Autodesk Inventor part; units mm, degrees
ref_plane "YZ Plane" through (0, 0, 0) normal (1, 0, 0) x (0, 1, 0)
ref_plane "XZ Plane" through (0, 0, 0) normal (0, 1, 0) x (-1, 0, 0)
ref_plane "XY Plane" through (0, 0, 0) normal (0, 0, 1) x (1, 0, 0)
sketch "Sketch1" plane through (0, 0, 0) normal (0, 0, 1) x (1, 0, 0)
  line L0 (6.4, 0) -> (7.6, 0)
  line L1 (12, -2.5403) -> (12, -5.8)
  line L2 (7.25, -6.4) -> (5, -6.4)
  line L3 (5, -6.4) -> (5, -16.4)
  line L4 (5, -16.4) -> (0, -16.4)
  line L5 (0, -16.4) -> (0, 0)
  line L6 (7.25, -6.4) -> (7.25, -5.8)
  line L7 (7.25, -5.8) -> (12, -5.8)
  line L8 (0, -1.28) -> (6.1, -1.28)
  line L9 (6.4, -0.98) -> (6.4, 0)
  line L10 (7.6, 0) -> (12, -2.5403)
  arc A0 (6.1, -1.28) -> (6.4, -0.98) centre (6.1, -0.98) ccw
  dimension "d0" = 24
  dimension "d1" = 10
  dimension "d3" = 10
  dimension "d4" = 14.5
  dimension "d5" = 0.6
  dimension "d26" = 15.2
  dimension "d27" = 30
  dimension "d28" = 12.8
  dimension "d29" = 1.28
  dimension "d30" = 0.3
  dimension "d31" = 6.4
revolve "Revolution1" add sketch "Sketch1" angle 360 about axis through (0, -16.4, 0) along (0, 1, 0)
sketch "Sketch2" plane through (0, 0, 0) normal (0, 1, 0) x (1, 0, 0)
  line L0 (0, -9.2376) -> (-8, -4.6188)
  line L1 (-8, -4.6188) -> (-8, 4.6188)
  line L2 (-8, 4.6188) -> (0, 9.2376)
  line L3 (0, 9.2376) -> (8, 4.6188)
  line L4 (8, 4.6188) -> (8, -4.6188)
  line L5 (8, -4.6188) -> (0, -9.2376)
  circle A0 centre (0, 0) radius 12
  point P0 (0, 0)
  point P1 (0, 0)
  dimension "d32" = 16
extrude "Extrusion1" cut sketch "Sketch2" against normal blind 5.8
thread "Thread1"
chamfer "Chamfer1" distance 0.8333 angle 45 1 edges at (-5, -16.4, 0)
equation "\"d0\" = 1.5 * S_"
equation "\"d1\" = d1_"
equation "\"d3\" = L"
equation "\"d4\" = dw"
equation "\"d5\" = hw"
equation "\"d26\" = 0.95 * S_"
equation "\"d28\" = 0.8 * S_"
equation "\"d29\" = 0.2 * k"
equation "\"d31\" = k"
equation "\"d14\" = b"
equation "\"d16\" = 0.0833333 * d"
equation "\"d32\" = S_"
equation "\"d33\" = k - hw"
equation "\"d1_\" = 10"
equation "\"S_\" = 16"
equation "\"k\" = 6.4"
equation "\"e\" = 17.6"
equation "\"L\" = 10"
equation "\"b\" = 8"
equation "\"Grip_Length\" = 2"
equation "\"dw\" = 14.5"
equation "\"hw\" = 0.6"
properties part number "Bolt 4A M10-6g×10(S16) GOST 7798-70" material "Steel, Mild"
Read the model definition and answer for the solid it produces. Units are mm, in the model's axes. A direction names the side the tool comes from. Coordinates: 2 decimals unless noted, no trailing zeros. Loops run counter-clockwise (first coordinate to the right, second up) from the corner with the lowest first, then second, coordinate; pieces in that order, holes last. Notation, with made-up numbers: (65.25, -23) -> (80.25, -23) arc R12 ccw to (80.25, -14) -> close; hole circle Ø5 at (33, -1.75). An arc over 180 degrees is marked (long way). Write item = value, one per line. Start each with the question number.
1) Given P1, Ø3.5, axis at x = 0, z = 2, coming from the +Y side; P2, Ø3, axis at y = -11, z = 2.5, coming from the -X side; P3, Ø1, axis at x = 4, y = -13, coming from the -Z side, each flat-ended and moving along its own axis, determine where each tip first touches the part or whether it passes through.
2) The part is cut by section B-B, the plane y = -5.5. Determine the outline of the cut face in (x, z), plus the area to 3 significant figures.
3) Find the intervals of material crossed by L1, parallel to X at y = -0.3, z = 0; L2, parallel to Y at x = 2.25, z = -2.25; L3, parallel to X at y = -6, z = 0.25, in increasing order. Write a range as from..to.
4) The part is cut by section A-A, the plane z = 0. Determine the outline of the cut face in (x, y), plus the area to 3 significant figures.
5) The part is cut by section C-C, the plane y = -14. Determine the outline of the cut face in (x, z).
6) The mould has two halves that part along X. Classify faces 1 (the face through (3.35, -6.1, 6.43)), 2 (the face through (-8, -3, 0)), 3 (the face through (-5.08, -0.48, 3.89)): pulls with the +X half, pulls with the -X half, needs draft (parallel to the pull), parting line crosses it, or undercut.
7) For faces 4 (the face through (-5, -5.8, -6)), 5 (the face through (3.944, -2.976, -6.961)), 6 (the face through (0, -1.28, 0)), determine the directions among +Z, -Z, +X, -X, +Y, -Y from which every point of the face is accessible in a straight line to the end or side of a thin tool.
Result:
q1.P1 = -1.28
q1.P2 = -4.9
q1.P3 = -3.57
q2.outline = (-8, -4.62) -> (0, -9.24) -> (8, -4.62) -> (8, 4.62) -> (0, 9.24) -> (-8, 4.62) -> close
q2.area = 222 mm²
q3.L1 = -8..-6.4, 6.4..8
q3.L2 = -16.4..-1.28
q3.L3 = -7.25..7.25
q4.outline = (-8, -5.8) -> (-7.25, -5.8) -> (-7.25, -6.4) -> (-5, -6.4) -> (-5, -15.57) -> (-4.17, -16.4) -> (4.17, -16.4) -> (5, -15.57) -> (5, -6.4) -> (7.25, -6.4) -> (7.25, -5.8) -> (8, -5.8) -> (8, -0.23) -> (7.6, 0) -> (6.4, 0) -> (6.4, -0.98) arc R0.3 cw to (6.1, -1.28) -> (-6.1, -1.28) arc R0.3 cw to (-6.4, -0.98) -> (-6.4, 0) -> (-7.6, 0) -> (-8, -0.23) -> close
q4.area = 184 mm²
q5.outline = circle Ø10 at (0, 0)
q6.face_1 = parting line crosses it
q6.face_2 = pulls with the -X half
q6.face_3 = undercut
q7.face_4 = -Y
q7.face_5 = -Z, +X, +Y, -Y
q7.face_6 = +Y
